Autodesk Inventor part; units mm, degrees
ref_plane "YZ Plane" through (0, 0, 0) normal (1, 0, 0) x (0, 1, 0)
ref_plane "XZ Plane" through (0, 0, 0) normal (0, 1, 0) x (-1, 0, 0)
ref_plane "XY Plane" through (0, 0, 0) normal (0, 0, 1) x (1, 0, 0)
sketch "Sketch1" plane through (0, 0, 0) normal (0, 1, 0) x (-1, 0, 0)
  line L0 (0, -110.6497) -> (0, 19.6497)
  line L1 (36.2497, 0) -> (-7.2497, 0)
  line L2 (5, 0) -> (24, 0)
  line L3 (29, -5) -> (29, -86)
  line L4 (24, -91) -> (5, -91)
  line L5 (0, -86) -> (0, -5)
  line L6 (0, 0) -> (29, -91) construction
  line L7 (29, 0) -> (0, -91) construction
  arc A0 (29, -5) -> (24, 0) centre (24, -5) ccw
  arc A1 (24, -91) -> (29, -86) centre (24, -86) ccw
  arc A2 (0, -86) -> (5, -91) centre (5, -86) ccw
  arc A3 (5, 0) -> (0, -5) centre (5, -5) ccw
  circle A4 centre (18, -8) radius 4
  circle A5 centre (18, -45.5) radius 3.5
  circle A6 centre (18, -83) radius 4
  point P0 (0, -5)
  dimension "d0" = 29
  dimension "d1" = 91
  dimension "d2" = 5
  dimension "d3" = 8
  dimension "d4" = 7
  dimension "d5" = 8
  dimension "d6" = 18
  dimension "d7" = 45.5
  dimension "d8" = 18
  dimension "d9" = 8
  dimension "d10" = 8
  dimension "d11" = 18
extrude "Extrusion1" add sketch "Sketch1" along normal blind 18 contours L0 A3 L1 A0 L3 A1 L4 A2 | A4 | A5 | A6
sketch "Sketch2" plane through (0, 0, -5) normal (1, 0, 0) x (0, 0, -1)
  line L0 (-5, -3.6) -> (-5, 21.6)
  line L1 (104.2, 0) -> (-23.2, 0)
  circle A0 centre (9, 14) radius 2.5
  line L2 (52, 10) -> (62, 10)
  line L3 (64, 8) -> (64, 5)
  line L4 (62, 3) -> (52, 3)
  line L5 (50, 5) -> (50, 8)
  line L6 (50, 10) -> (64, 3) construction
  line L7 (64, 10) -> (50, 3) construction
  arc A1 (64, 8) -> (62, 10) centre (62, 8) ccw
  arc A2 (62, 3) -> (64, 5) centre (62, 5) ccw
  arc A3 (50, 5) -> (52, 3) centre (52, 5) ccw
  arc A4 (52, 10) -> (50, 8) centre (52, 8) ccw
  point P0 (-5, 0)
  point P1 (57, 6.5)
  point P2 (50, 6.5)
  dimension "d14" = 5
  dimension "d15" = 14
  dimension "d16" = 14
  dimension "d17" = 14
  dimension "d18" = 7
  dimension "d19" = 2
  dimension "d20" = 55
  dimension "d21" = 3
extrude "Extrusion2" cut sketch "Sketch1" along normal blind 2 contours A4 | A5 | A6
extrude "Extrusion3" cut sketch "Sketch2" against normal blind 8
properties part number "camera_model"
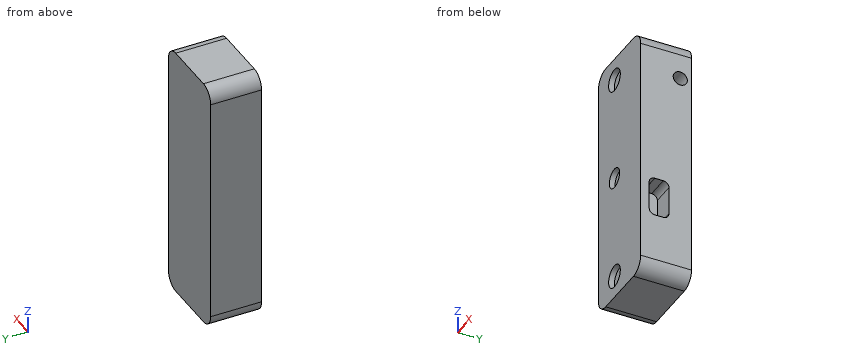
Geometry check sheet. Reference: the model listing, model coordinates, mm. Round coordinates to 2 decimals unless told otherwise and drop trailing zeros. Loops run counter-clockwise (first coordinate to the right, second up) from the corner with the lowest first, then second, coordinate; pieces in that order, holes last. Notation, with made-up numbers: (70.25, 46.5) - (80.25, 46.5) arc R31 ccw to (80.25, 75.5) - close; hole circle Ø2 at (34.5, 68). An arc over 180 degrees is marked (long way). One line per question, with ' | ' between items. Start each with the question number.
1. Depth check by flat-ended pin: pin 1 (2.5 mm diameter, centred on x = -19, z = -9.5, fed in from -Y); pin 2 (3 mm diameter, centred on y = 14, z = -14, fed in from +X); pin 3 (1.5 mm diameter, centred on x = -2.5, y = 7, fed in from -Z). Enter the tip coordinate at first touch or a pass-through.
2. Cross-section at C-C on y = 12.5. Record the cut outline in (x, z), then the cut area to 3 significant figures.
3. Cross-section at B-B on x = -18. Record the cut outline in (y, z).
4. Scan lines: line 1 (Z direction, x = -18, y = 0.7); line 2 (Y direction, x = -2.75, z = -14); line 3 (Y direction, x = -7, z = -65). Record each from-to range of solid material in increasing order. Write a range as [from, to].
5. Cross-section at A-A on z = -83. Record the cut outline in (x, y), then the cut area to 3 significant figures.
6. Cross-section at D-D on x = -1.75. Record the cut outline in (y, z), then the cut area to 3 significant figures.
Taken from the geometry:
1) pin 1: y = 2 | pin 2: x = -8 | pin 3: z = -90.68
2) outline: (-29, -86) arc R5 ccw to (-24, -91) - (-5, -91) arc R5 ccw to (0, -86) - (0, -16) - (-8, -16) - (-8, -12) - (0, -12) - (0, -5) arc R5 ccw to (-5, 0) - (-24, 0) arc R5 ccw to (-29, -5) - close | area: 2,590 mm²
3) outline: (0, -91) - (18, -91) - (18, 0) - (0, 0) - (0, -4) - (2, -4) - (2, -12) - (0, -12) - (0, -42) - (2, -42) - (2, -49) - (0, -49) - (0, -79) - (2, -79) - (2, -87) - (0, -87) - close
4) line 1: [-91, -87], [-79, -49], [-42, -12], [-4, 0] | line 2: [0, 11.5], [16.5, 18] | line 3: [0, 3], [10, 18]
5) outline: (-29, 0) - (-22, 0) - (-22, 2) - (-14, 2) - (-14, 0) - (0, 0) - (0, 18) - (-29, 18) - close | area: 506 mm²
6) outline: (0, -89.8) - (18, -89.8) - (18, -1.2) - (0, -1.2) - close; hole (3, -67) arc R2 ccw to (5, -69) - (8, -69) arc R2 ccw to (10, -67) - (10, -57) arc R2 ccw to (8, -55) - (5, -55) arc R2 ccw to (3, -57) - close; hole circle Ø5 at (14, -14) | area: 1,480 mm²
